For this review, take the finished solid that the model builds, in its own axes (mm). Coordinates: 2 decimals unless noted, no trailing zeros. Order: outer loops, then holes, each group sorted by start corner. A loop starts at its lowest first (then second) coordinate and runs counter-clockwise, first axis right, second up. Notation, with made-up numbers: (39.5, 55) -> (92.5, 55) arc R10 cw to (92.5, 66) -> close; hole circle Ø5 at (6.25, -38.75). An arc over 180 degrees is marked (long way). Answer as a JSON object with one key per item and string values. Group by question number.
1) For pin 1 (4 mm diameter, centred on y = -7, z = 50.5, fed in from +X), flat-tipped, find the tip position at first contact; note if it passes through.
2) Add section B-B, the plane x = -1.7. Write out the cut boundary in (y, z).
3) Wall thickness on L1, parallel to Y at x = -1.1, z = 17; L2, parallel to Y at x = -1.25, z = 55: over which ranges is each line inside the solid? List them lowest first.
4) Add section A-A, the plane z = 116. Write out the cut boundary in (x, y).
from build123d import *

# Parameters (mm, degrees)
SKETCH1_W           = 2
SKETCH1_H           = 40
BOSS_EXTRUDE1_DEPTH = 165
CUT_EXTRUDE1_DEPTH  = 165
CUT_EXTRUDE2_DEPTH  = 165


with BuildPart() as part:
    # Sketch1 → Boss-Extrude1 (new body)
    with BuildSketch(Plane.XY):
        with Locations((-1, -17.620909594)):
            Rectangle(SKETCH1_W, SKETCH1_H)
    extrude(amount=BOSS_EXTRUDE1_DEPTH)

    # Sketch2 → Cut-Extrude1 (cut)
    with BuildSketch(Plane.XY.offset(165)):
        Polygon((0, 2.379090406), (-1, 2.379090406), (0, 0), align=None)
    extrude(amount=-CUT_EXTRUDE1_DEPTH, mode=Mode.SUBTRACT)

    # Sketch3 → Cut-Extrude2 (cut)
    with BuildSketch(Plane.XY.offset(165)):
        Polygon((-1, 2.379090406), (-2, 2.379090406), (-2, 0), align=None)
    extrude(amount=-CUT_EXTRUDE2_DEPTH, mode=Mode.SUBTRACT)


solid = part.part
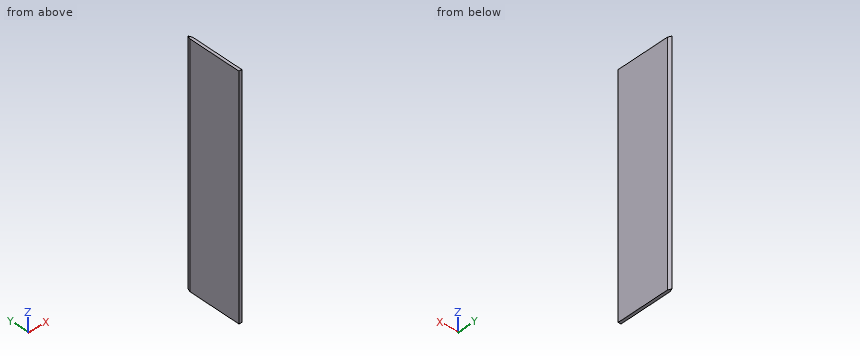
Output values:
{
 "1": {"pin 1": "stops at x = 0"},
 "2": {"outline": "(-37.62, 0) -> (0.71, 0) -> (0.71, 165) -> (-37.62, 165) -> close"},
 "3": {"L1": "y = -37.62 to 2.14", "L2": "y = -37.62 to 1.78"},
 "4": {"outline": "(-2, -37.62) -> (0, -37.62) -> (0, 0) -> (-1, 2.38) -> (-2, 0) -> close"}
}
